CAD build for the part. Positions are in the model's coordinates, mm. A direction names the side the tool comes from. Give positions to 0.01 mm unless a question says otherwise; leave off trailing zeros. Write each loop counter-clockwise with the first axis right and the second up, starting at its lowest first coordinate (ties: lowest second). Pieces come first, ordered by that corner, then holes. Notation, with made-up numbers: (20.25, 59) - (70.25, 59) arc R17 ccw to (70.25, 88) - close; hole circle Ø1 at (31, 85). An arc over 180 degrees is marked (long way). Put each result on its own line as item: value. Start each with the question number.
1. Cut at B-B on z = 0. List the corners of the cut face in (x, y).
2. Cut at C-C on y = 0.8. List the corners of the cut face in (x, z).
3. Cut at D-D on x = 11. List the corners of the cut face in (y, z), and give its area (3 significant figures).
4. Wall check: line 1 (Z direction, x = -6.5, y = 0.35); line 2 (Z direction, x = -14, y = -0.4); line 3 (Z direction, x = 21, y = 0.4). Give the ranges that are in metal, low to high.
5. Cut at A-A on x = -14. List the corners of the cut face in (y, z).
6. Drop flat-ended pins along their axis: pin 1 (1 mm diameter, centred on x = -15.5, y = 0, fed in from -Z) (3 decimals); pin 2 (5 mm diameter, centred on x = -29, z = 0, fed in from +Y); pin 3 (0.5 mm diameter, centred on x = -3, y = 0.5, fed in from +Z); pin 4 (1 mm diameter, centred on x = 23, y = 0, fed in from -Z). Give the stop position or say it passes through.
7. Tool access for faces 1 (the flat face through (22, 0, -5.215)), 2 (the flat face through (-2.978, 0, 0)), 3 (the cylindrical face through (31.213, 0.024, 0.115)): list every direction of +Z, -Z, +X, -X, +Y, -Y with a clear straight run to the whole face (end or side of a thin tool).
8. Mould opens along X. For faces 4 (the cylindrical face through (-6.292, 0.024, -11.404)), 5 (the cylindrical face through (-33.99, 0.02, -0.69)), 6 (the flat face through (21, 0, 5.215)) say: +X half, -X half, draft (parallel to the pull), parting line (faces both ways), or undercut.
from build123d import *

# Parameters (mm, degrees)
SKETCH1_W           = 70
SKETCH1_H           = 3.5
BOSS_EXTRUDE1_DEPTH = 25
SKETCH2_R           = 10.1
SKETCH2_R_2         = 1.6
CUT_EXTRUDE1_DEPTH  = 44.153794735
SKETCH4_OUTSIDE_W   = 89.218
SKETCH4_OUTSIDE_H   = 69.218
CUT_EXTRUDE2_DEPTH  = 44.153794735
SKETCH5_W           = 1
SKETCH5_H           = 2.5
CUT_EXTRUDE3_DEPTH  = 40.601136347
CHAMFER1_SIZE       = 0.460537939
CHAMFER1_SIZE_2     = 0.4


with BuildPart() as part:
    # Sketch1 → Boss-Extrude1 (new, symmetric)
    with BuildSketch(Plane.XY):
        Rectangle(SKETCH1_W, SKETCH1_H)
    extrude(amount=BOSS_EXTRUDE1_DEPTH, both=True)

    # Sketch2 → Cut-Extrude1 (cut, through all)
    with BuildSketch(Plane(origin=(0, 1.75, 0), x_dir=(1, 0, 0), z_dir=(0, 1, 0))):
        with Locations(Location((-14, 0, 0), (0, 0, 180))):
            Circle(SKETCH2_R)
        with Locations((-29, 0)):
            Circle(SKETCH2_R_2)
        with Locations(Location((-6.5, 12.990381057, 0), (0, 0, 180))):
            Circle(SKETCH2_R_2)
        with Locations(Location((-6.5, -12.990381057, 0), (0, 0, 180))):
            Circle(SKETCH2_R_2)
        with Locations(Location((11, 0, 0), (0, 0, 180))):
            Circle(SKETCH2_R_2)
        with Locations(Location((26, 0, 0), (0, 0, 180))):
            Circle(SKETCH2_R_2)
    extrude(amount=-CUT_EXTRUDE1_DEPTH, mode=Mode.SUBTRACT)

    # Sketch4 outside → Cut-Extrude2 (cut, through all)
    with BuildSketch(Plane(origin=(0, 1.75, 0), x_dir=(1, 0, 0), z_dir=(0, 1, 0))):
        Rectangle(SKETCH4_OUTSIDE_W, SKETCH4_OUTSIDE_H)
        with BuildLine():
            Line((17.054712149, -5.214702174), (26, -5.214702174))
            ThreePointArc((26, -5.214702174), (31.214702174, 0), (26, 5.214702174))
            Line((26, 5.214702174), (17.054712149, 5.214702174))
            ThreePointArc((17.054712149, 5.214702174), (8.454737914, 7.157470503), (1.525041378, 12.608453125))
            ThreePointArc((1.525041378, 12.608453125), (-34, 0), (1.525041378, -12.608453125))
            ThreePointArc((1.525041378, -12.608453125), (8.454737914, -7.157470503), (17.054712149, -5.214702174))
        make_face(mode=Mode.SUBTRACT)
    extrude(amount=-CUT_EXTRUDE2_DEPTH, mode=Mode.SUBTRACT)

    # Sketch5 → Cut-Extrude3 (cut, through all)
    with BuildSketch(Plane(origin=(0, 1.75, 0), x_dir=(1, 0, 0), z_dir=(0, 1, 0))):
        with Locations((-3.477649976, 0)):
            Rectangle(SKETCH5_W, SKETCH5_H)
    extrude(amount=-CUT_EXTRUDE3_DEPTH, mode=Mode.SUBTRACT)

    # Chamfer1
    # the kernel refuses this chamfer: 0.460537939, 0.4 mm, written as the material it takes off along each edge
    with BuildSketch(Plane(origin=(-3.977649976, 2.93802649, 1.25), x_dir=(1, 0, 0), z_dir=(0, -1, 0))) as chamfer1_piece_1:
        with BuildLine():
            Line((CHAMFER1_SIZE, 0), (-0.058717526, 0.404094149))
            ThreePointArc((-0.058717526, 0.404094149), (-0.028274639, 0.208923305), (0, 0))
            Line((0, 0), (CHAMFER1_SIZE, 0))
        make_face()
    extrude(amount=5.876052981, mode=Mode.SUBTRACT)
    with BuildSketch(Plane(origin=(-3.977649976, 2.974865586, -1.25), x_dir=(-0.1470633692519934, 0, -0.9891270724352114), z_dir=(0, -1, 0))) as chamfer1_piece_2:
        with BuildLine():
            Line((0.475023444, 0), (-CHAMFER1_SIZE_2 * 0.147063369252, CHAMFER1_SIZE_2 * 0.989127072435))
            Line((-CHAMFER1_SIZE_2 * 0.147063369252, CHAMFER1_SIZE_2 * 0.989127072435), (0, 0))
            ThreePointArc((0, 0), (0.244917786, 0.002790335), (0.475023444, 0))
        make_face()
    extrude(amount=5.949731171, mode=Mode.SUBTRACT)
    # the kernel refuses this chamfer: 0.460537939, 0.4 mm, written as the material it takes off along each edge
    with BuildSketch(Plane(origin=(-14, -1.75, 0), x_dir=(0.9980739544649045, 0, 0.062035323959722194), z_dir=(0.062035323959722194, 0, -0.9980739544649045))) as chamfer1_2_piece_1:
        Polygon((10.1 + CHAMFER1_SIZE_2, 0), (10.1, -CHAMFER1_SIZE_2), (10.1, 0), align=None)
    revolve(axis=Axis((-14, -1.75, 0), (0, -1, 0)), revolution_arc=352.508320322, mode=Mode.SUBTRACT)
    with BuildSketch(Plane(origin=(-14, 1.75, 0), x_dir=(0.9980739544649045, 0, 0.06203532395972309), z_dir=(0.06203532395972309, 0, -0.9980739544649045))) as chamfer1_2_piece_2:
        Polygon((10.1 + CHAMFER1_SIZE_2, 0), (10.1, CHAMFER1_SIZE_2), (10.1, 0), align=None)
    revolve(axis=Axis((-14, 1.75, 0), (0, -1, 0)), revolution_arc=352.508320322, mode=Mode.SUBTRACT)


solid = part.part
Report:
1. outline: (-34, -1.75) - (-30.6, -1.75) - (-30.6, 1.75) - (-34, 1.75) - close; (-27.4, -1.75) - (-24.5, -1.75) - (-24.1, -1.35) - (-24.1, 1.35) - (-24.5, 1.75) - (-27.4, 1.75) - close; (-2.98, -1.75) - (9.4, -1.75) - (9.4, 1.75) - (-2.98, 1.75) - close; (12.6, -1.75) - (24.4, -1.75) - (24.4, 1.75) - (12.6, 1.75) - close; (27.6, -1.75) - (31.21, -1.75) - (31.21, 1.75) - (27.6, 1.75) - close
2. outline: (1.53, -12.61) arc R20.01 cw to (17.05, -5.21) - (26, -5.21) arc R5.21 ccw to (26, 5.21) - (17.05, 5.21) arc R20.01 cw to (1.53, 12.61) arc R20 ccw (long way) to start; hole circle Ø3.2 at (-29, 0); hole circle Ø3.2 at (-6.5, -12.99); hole circle Ø3.2 at (-6.5, 12.99); hole (-4.05, -1.72) - (-3.58, -1.25) - (-2.98, -1.25) - (-2.98, 1.25) - (-3.52, 1.25) - (-4.04, 1.65) arc R10.1 ccw (long way) to start; hole circle Ø3.2 at (11, 0); hole circle Ø3.2 at (26, 0)
3. outline: (-1.75, -6.15) - (1.75, -6.15) - (1.75, -1.6) - (-1.75, -1.6) - close; (-1.75, 1.6) - (1.75, 1.6) - (1.75, 6.15) - (-1.75, 6.15) - close
3. area: 31.9 mm²
4. line 1: z = -18.54 to -14.59, -11.39 to -6.76, 6.76 to 11.39, 14.59 to 18.54
4. line 2: z = -20 to -10.1, 10.1 to 20
4. line 3: z = -5.21 to 5.21
5. outline: (-1.75, -20) - (1.75, -20) - (1.75, -10.5) - (1.35, -10.1) - (-1.35, -10.1) - (-1.75, -10.5) - close; (-1.75, 10.5) - (-1.35, 10.1) - (1.35, 10.1) - (1.75, 10.5) - (1.75, 20) - (-1.75, 20) - close
6. pin 1: stops at z = -19.975
6. pin 2: stops at y = 1.75
6. pin 3: stops at z = 16.87
6. pin 4: stops at z = -5.21
7. face 1: -Z, +X, +Y, -Y
7. face 2: +Y, -Y
7. face 3: +X, +Y, -Y
8. face 4: undercut
8. face 5: parting line
8. face 6: draft
